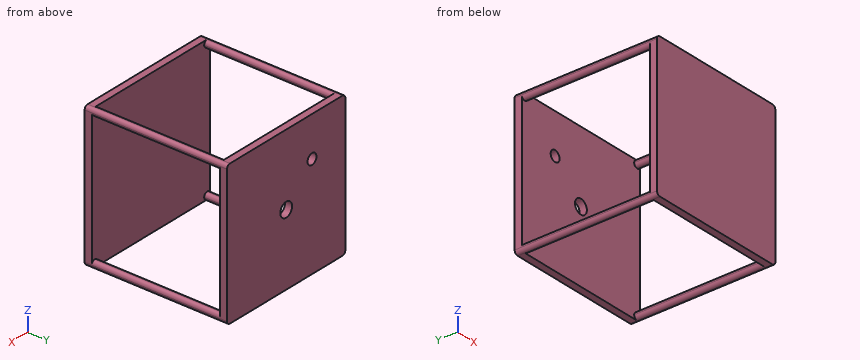
```python
from build123d import *

# Parameters (mm, degrees)
SKETCH2_W           = 400
SKETCH2_H           = 400
BOSS_EXTRUDE1_DEPTH = 400
SKETCH3_W           = 360
SKETCH3_H           = 360
CUT_EXTRUDE4_DEPTH  = 400
SKETCH5_W           = 360
SKETCH5_H           = 360
CUT_EXTRUDE5_DEPTH  = 400
FILLET1_R           = 10
FILLET2_START       = -1
FILLET2_DEPTH       = 402
FILLET3_R           = 10
FILLET4_R           = 10
FILLET6_R           = 10
FILLET7_R           = 10
FILLET8_R           = 10
SKETCH6_R           = 20
CUT_EXTRUDE6_DEPTH  = 20
SKETCH9_R           = 15
CUT_EXTRUDE8_DEPTH  = 71


with BuildPart() as part:
    # Sketch2 → Boss-Extrude1 (new body)
    with BuildSketch(Plane(origin=(0, 0, 0), x_dir=(1, 0, 0), z_dir=(0, 1, 0))):
        Rectangle(SKETCH2_W, SKETCH2_H)
    extrude(amount=BOSS_EXTRUDE1_DEPTH)

    # Sketch3 → Cut-Extrude4 (cut)
    with BuildSketch(Plane.XY.offset(200)):
        with Locations((0, 200)):
            Rectangle(SKETCH3_W, SKETCH3_H)
    extrude(amount=-CUT_EXTRUDE4_DEPTH, mode=Mode.SUBTRACT)

    # Sketch5 → Cut-Extrude5 (cut)
    with BuildSketch(Plane.ZY.offset(200)):
        with Locations((0, 200)):
            Rectangle(SKETCH5_W, SKETCH5_H)
    extrude(amount=-CUT_EXTRUDE5_DEPTH, mode=Mode.SUBTRACT)

    # Fillet1
    fillet1_edges = [part.edges().sort_by_distance(p)[0] for p in [
        (200, 200, 180),
    ]]
    fillet(fillet1_edges, radius=FILLET1_R)

    # Fillet2: read off the stored shape, not the designer's step
    # Fillet2 outline → Fillet2 (cut)
    with BuildSketch(Plane(origin=(0, 0, 0), x_dir=(1, 0, 0), z_dir=(0, 1, 0)).offset(FILLET2_START)):
        with BuildLine():
            Line((200, -200), (200, -190))
            ThreePointArc((200, -190), (197.071067812, -197.071067812), (190, -200))
            Line((190, -200), (200, -200))
        make_face()
    extrude(amount=FILLET2_DEPTH, mode=Mode.SUBTRACT)

    # Fillet3
    fillet3_edges = [part.edges().sort_by_distance(p)[0] for p in [
        (180, 200, 180),
    ]]
    fillet(fillet3_edges, radius=FILLET3_R - 0.0001)  # a hair under: the kernel refuses the full size

    # Fillet4
    fillet4_edges = [part.edges().sort_by_distance(p)[0] for p in [
        (180, 200, 200),
    ]]
    fillet(fillet4_edges, radius=FILLET4_R - 0.0001)  # a hair under: the kernel refuses the full size

    # Fillet6
    fillet6_edges = [part.edges().sort_by_distance(p)[0] for p in [
        (-180, 200, -180),
        (-180, 200, -200),
        (-200, 200, -200),
        (-200, 200, -180),
    ]]
    fillet(fillet6_edges, radius=FILLET6_R - 0.0001)  # a hair under: the kernel refuses the full size

    # Fillet7
    fillet7_edges = [part.edges().sort_by_distance(p)[0] for p in [
        (200, 200, -180),
        (180, 200, -180),
        (180, 200, -200),
        (200, 200, -200),
    ]]
    fillet(fillet7_edges, radius=FILLET7_R - 0.0001)  # a hair under: the kernel refuses the full size

    # Fillet8
    fillet8_edges = [part.edges().sort_by_distance(p)[0] for p in [
        (-180, 200, 180),
        (-200, 200, 180),
        (-180, 200, 200),
        (-200, 200, 200),
    ]]
    fillet(fillet8_edges, radius=FILLET8_R - 0.0001)  # a hair under: the kernel refuses the full size

    # Sketch6 → Cut-Extrude6 (cut)
    with BuildSketch(Plane(origin=(0, 400, 0), x_dir=(1, 0, 0), z_dir=(0, 1, 0))):
        with Locations(Location((0, 0, 0), (0, 0, 270))):
            Circle(SKETCH6_R)
    extrude(amount=-CUT_EXTRUDE6_DEPTH, mode=Mode.SUBTRACT)

    # Sketch9 → Cut-Extrude8 (cut)
    with BuildSketch(Plane(origin=(0, 400, 0), x_dir=(1, 0, 0), z_dir=(0, 1, 0))):
        with Locations(Location((-87.327687477, -87.327687477, 0), (0, 0, 270))):
            Circle(SKETCH9_R)
    extrude(amount=-CUT_EXTRUDE8_DEPTH, mode=Mode.SUBTRACT)


solid = part.part
```
Geometry: final body of the model. Coordinates: model frame, mm. Coordinates: 2 decimals unless noted, no trailing zeros. Write each loop counter-clockwise with the first axis right and the second up, starting at its lowest first coordinate (ties: lowest second). Pieces come first, ordered by that corner, then holes. Notation, with made-up numbers: M 13.5,14 L 31.5,14 A12 ccw 31.5,22 Z; hole C 6.25,34 d7. An arc over 180 degrees is marked long. Answer as CSV lines item,"result". Start each with the question number.
Q1. Cut plane C-C on x = -40.5. Return the cut outline in (y, z).
Q2. Line query: line 1 (Y direction, x = 69.5, z = 107); line 2 (X direction, y = 395, z = 0); line 3 (Y direction, x = -77.5, z = 88). Output: solid intervals per line, ascending. Write a range as from..to.
Q3. Cut plane A-A on z = 0. Return the cut outline in (x, y), then the cut area to 3 significant figures.
Q4. Cut plane B-B on y = 71. Count the separate pieces of the cut face and the enclosed holes in it, then the cut area to 3 significant figures.
Q5. Cut plane D-D on z = -113. Return the cut outline in (x, y).
Findings below:
1,outline,"M 0,-200 L 20,-200 L 20,200 L 0,200 Z; M 380,-200 L 400,-200 L 400,200 L 380,200 Z"
2,line 1,"y = 0..20, 380..400"
2,line 2,"x = -200..-20, 20..200"
2,line 3,"y = 0..20"
3,outline,"M -200,0 L 200,0 L 200,20 L -200,20 Z; M -200,380 L -20,380 L -20,400 L -200,400 Z; M 20,380 L 200,380 L 200,400 L 20,400 Z"
3,area,"15,200 mm2"
4,separate pieces,"4"
4,enclosed holes,"0"
4,area,"1,260 mm2"
5,outline,"M -200,0 L 200,0 L 200,20 L -200,20 Z; M -200,380 L 200,380 L 200,400 L -200,400 Z"
